Autodesk Fusion 360 part; units mm, degrees
sketch "Sketch1" plane through (0, 0, 0) normal (0, 0, 1) x (1, 0, 0)
  line L0 (0, 0) -> (82.25, 0)
  line L1 (82.25, 0) -> (82.25, 89.5)
  line L2 (82.25, 89.5) -> (0, 89.5)
  line L3 (0, 89.5) -> (0, 0)
  dimension "d1" = 89.5
  dimension "d2" = 82.25
extrude "Extrude1" add sketch "Sketch1" along normal blind 8.5
shell "Shell1" thickness 2 removed faces 1 at (27.4167, 59.6667, 8.5)
fillet "Fillet1" radius 3 8 edges at (0, 0, 4.25) (82.25, 0, 4.25) (82.25, 89.5, 4.25) (0, 89.5, 4.25) (41.125, 89.5, 0) (0, 44.75, 0) (41.125, 0, 0) (82.25, 44.75, 0)
chamfer "Chamfer1" distance 0.5 angle 45 4 edges at (2, 44.75, 8.5) (41.125, 2, 8.5) (41.125, 87.5, 8.5) (80.25, 44.75, 8.5)
equation "d1 = 85.5 mm + 4 mm"
equation "d2 = 78.25 mm + 4 mm"
equation "d3 = 6.5 mm + 2 mm"
For this review, take the finished solid that the model builds, in its own axes (mm). A direction names the side the tool comes from. Round coordinates to 2 decimals unless told otherwise and drop trailing zeros. Write each loop counter-clockwise with the first axis right and the second up, starting at its lowest first coordinate (ties: lowest second). Pieces come first, ordered by that corner, then holes. Notation, with made-up numbers: M 28.25,38.25 L 42.25,38.25 A21 ccw 42.25,74.25 Z; hole C 73.5,-4 d1. An arc over 180 degrees is marked long. One line per item, written item: value. Start each with the question number.
(1) Insertion check: pin 1 (10 mm diameter, centred on x = 29.5, y = 48.5, fed in from +Z); pin 2 (4 mm diameter, centred on y = 14.5, z = 1, fed in from -X). Each pin has a flat end and moves straight along its axis. Give the tip position at first contact, or say it passes through.
(2) We need section C-C (x = 27). Give the boundary of the cut face in (y, z).
(3) Wall thickness on line 1 (X direction, y = 47.5, z = 3.5); line 2 (Y direction, x = 72, z = 6.5); line 3 (Z direction, x = 36.5, y = 44): over which ranges is each line inside the solid? List them lowest first.
(4) Machinability: for faces 4 (the flat face through (2, 45, 5)), 5 (the cylindrical face through (0.86, 44.17, 0.9)), which of the approach directions +Z, -Z, +X, -X, +Y, -Y give a long, thin tool a straight path to every point of the face, cutting with its end or side? Answer none if there is none.
(5) The part is to be moulded in two halves that separate along Y. For faces 1 (the flat face through (42, 87.5, 5)), 2 (the flat face through (82.25, 44, 6)), 3 (the flat face through (41, 0, 6)), say which applies: released by +Y, released by -Y, zero draft, split by the parting line, or undercut.
(6) We need section B-B (y = 43). Give the boundary of the cut face in (x, z), and give its area (3 significant figures).
(7) We need section A-A (z = 4). Give the boundary of the cut face in (x, y).
Result:
1. pin 1: z = 2
1. pin 2: x = 0
2. outline: M 0,3 A3 ccw 3,0 L 86.5,0 A3 ccw 89.5,3 L 89.5,8.5 L 88,8.5 L 87.5,8 L 87.5,2 L 2,2 L 2,8 L 1.5,8.5 L 0,8.5 Z
3. line 1: 0 to 2, 80.25 to 82.25
3. line 2: 0 to 2, 87.5 to 89.5
3. line 3: 0 to 2
4. face 4: +Z
4. face 5: -Z, -X, +Y, -Y
5. face 1: undercut
5. face 2: zero draft
5. face 3: released by -Y
6. outline: M 0,3 A3 ccw 3,0 L 79.25,0 A3 ccw 82.25,3 L 82.25,8.5 L 80.75,8.5 L 80.25,8 L 80.25,2 L 2,2 L 2,8 L 1.5,8.5 L 0,8.5 Z
6. area: 186 mm²
7. outline: M 0,3 A3 ccw 3,0 L 79.25,0 A3 ccw 82.25,3 L 82.25,86.5 A3 ccw 79.25,89.5 L 3,89.5 A3 ccw 0,86.5 Z; hole M 2,2 L 80.25,2 L 80.25,87.5 L 2,87.5 Z
